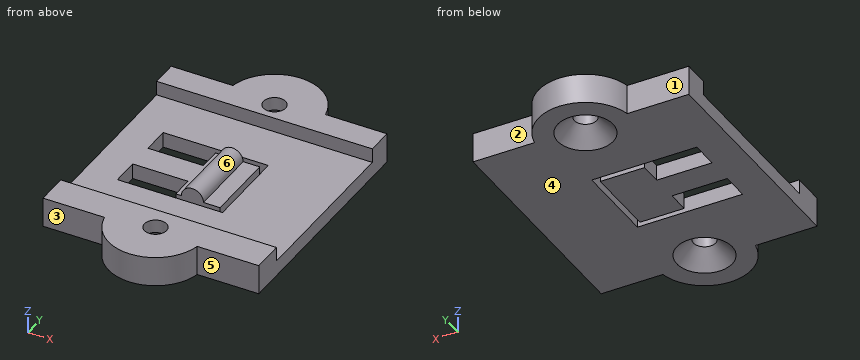
```python
from build123d import *

# Parameters (mm, degrees)
F1_DEPTH       = 5.4
F2_W           = 31.4
F2_H           = 2.6
F3_DEPTH       = 40
F4_W           = 2
F4_H           = 13
F6_D           = 4
F6_CSINK_D     = 10
F6_CSINK_ANGLE = 90


with BuildPart() as f1:
    # F0 (on Top) → F1 (new body)
    with BuildSketch(Plane.XY):
        with BuildLine():
            ThreePointArc((19.5610458605, 16.0277770907), (11.1944455951, 23.0277770907), (2.8278453298, 16.0277770907))
            Line((2.8278453298, 16.0277770907), (19.5610458605, 16.0277770907))
        make_face()
        with BuildLine():
            Line((19.5610458605, -25.9722229093), (2.8278453298, -25.9722229093))
            ThreePointArc((2.8278453298, -25.9722229093), (11.1944455951, -32.9722229093), (19.5610458605, -25.9722229093))
        make_face()
        with BuildLine():
            Line((2.8278453298, 16.0277770907), (-8.3055544049, 16.0277770907))
            Line((-8.3055544049, 16.0277770907), (-8.3055544049, -25.9722229093))
            Line((-8.3055544049, -25.9722229093), (2.8278453298, -25.9722229093))
            ThreePointArc((2.8278453298, -25.9722229093), (10.4414855216, -16.0056385255), (19.6944455951, -24.4722229093))
            ThreePointArc((19.6944455951, -24.4722229093), (19.6610299789, -25.2251829828), (19.5610458605, -25.9722229093))
            Line((19.5610458605, -25.9722229093), (30.6944455951, -25.9722229093))
            Line((30.6944455951, -25.9722229093), (30.6944455951, 16.0277770907))
            Line((30.6944455951, 16.0277770907), (19.5610458605, 16.0277770907))
            ThreePointArc((19.5610458605, 16.0277770907), (19.6610299789, 15.2807371642), (19.6944455951, 14.5277770907))
            ThreePointArc((19.6944455951, 14.5277770907), (10.4414855216, 6.0611927069), (2.8278453298, 16.0277770907))
        make_face()
        Polygon((7.6944455951, -7.4722229093), (7.6944455951, -2.4722229093), (-2.3055544049, -2.4722229093), (-2.3055544049, 2.5277770907), (7.6944455951, 2.5277770907), (16.6944455951, 2.5277770907), (16.6944455951, 1.5277770907), (16.6944455951, -11.4722229093), (16.6944455951, -12.4722229093), (7.6944455951, -12.4722229093), (-2.3055544049, -12.4722229093), (-2.3055544049, -7.4722229093), align=None, mode=Mode.SUBTRACT)
        with BuildLine():
            ThreePointArc((19.6944455951, -24.4722229093), (10.4414855216, -16.0056385255), (2.8278453298, -25.9722229093))
            Line((2.8278453298, -25.9722229093), (19.5610458605, -25.9722229093))
            ThreePointArc((19.5610458605, -25.9722229093), (19.6610299789, -25.2251829828), (19.6944455951, -24.4722229093))
        make_face()
        with BuildLine():
            Line((19.5610458605, 16.0277770907), (2.8278453298, 16.0277770907))
            ThreePointArc((2.8278453298, 16.0277770907), (10.4414855216, 6.0611927069), (19.6944455951, 14.5277770907))
            ThreePointArc((19.6944455951, 14.5277770907), (19.6610299789, 15.2807371642), (19.5610458605, 16.0277770907))
        make_face()
        Polygon((15.6944455951, 1.5277770907), (7.6944455951, 1.5277770907), (7.6944455951, -2.4722229093), (7.6944455951, -7.4722229093), (7.6944455951, -11.4722229093), (15.6944455951, -11.4722229093), align=None)
    extrude(amount=F1_DEPTH)

    # F2 (on face) → F3 (cut)
    with BuildSketch(Plane.YZ.offset(30.6944455951)):
        with Locations((-4.4722229093, 4.1)):
            Rectangle(F2_W, F2_H)
    extrude(amount=-F3_DEPTH, mode=Mode.SUBTRACT)

    # F4 (on face) → F5 (revolve)
    with BuildSketch(Plane.XY.offset(2.8)):
        with Locations((9.6944455951, -4.9722229093)):
            Rectangle(F4_W, F4_H)
    revolve(axis=Axis((10.6944455951, -4.9722229093, 2.8), (0, 1, 0)))

    # F6 (through all)
    with Locations(Plane(origin=(0, 0, 0), x_dir=(1, 0, 0), z_dir=(0, 0, -1))):
        with Locations((11.1944455951, 24.4722229093), (11.1944455951, -14.5277770907)):
            CounterSinkHole(F6_D / 2, F6_CSINK_D / 2, counter_sink_angle=F6_CSINK_ANGLE)


solid = f1.part
```
Read the model definition and answer for the solid it produces. Units are mm, in the model's axes. Face numbers are marked on the shaded views. A direction names the side the tool comes from. Round coordinates to 2 decimals unless told otherwise and drop trailing zeros. Write each loop counter-clockwise with the first axis right and the second up, starting at its lowest first coordinate (ties: lowest second). Pieces come first, ordered by that corner, then holes. Notation, with made-up numbers: (-3.5, 28.25) - (1.5, 28.25) arc R27 cw to (1.5, 64.25) - close; hole circle Ø4 at (-17, 85.5). An arc over 180 degrees is marked (long way). One line per item, written item: value.
Q1. Which of the six approach directions +Z, -Z, +X, -X, +Y, -Y give full straight-line access (tool end or side, diameter ignored) to the marked faces 1, 2 and 3?
The answers:
face 1: +Z, -Z, -X, +Y
face 2: +Z, -Z, +X, +Y
face 3: +Z, -Z, -X, -Y
Q2. For a pull along Y with two mould halves and no side action, classify the marked faces 4, 5 and 6 as pulls with the +Y half, pulls with the -Y half, needs draft (parallel to the pull), parting line crosses it, or undercut.
The answers:
face 4: needs draft
face 5: pulls with the -Y half
face 6: undercut
Q3. Straight lines are drawn through the part: line 1 (Y direction, x = 2.5, z = 0.4); line 2 (Y direction, x = -4, z = 4.1); line 3 (Y direction, x = 9, z = 0.65). For each, find the intervals that lie inside material, in ascending order. Write a range as from..to.
The answers:
line 1: y = -25.97..-12.47, -7.47..-2.47, 2.53..16.03
line 2: y = -25.97..-20.17, 11.23..16.03
line 3: y = -32.68..-28.23, -20.72..-12.47, -11.47..1.53, 2.53..10.77, 18.28..22.74
Q4. Each of these flat-tipped pins is pushed along its axis until it touches: P1, Ø1, axis at x = 7, y = -13.5, coming from the +Z side; P2, Ø1.6, axis at x = 26, z = 3.5, coming from the +Y side; P3, Ø3, axis at x = 3.5, z = 1, coming from the -Y side. Where does it stop, or does it pass through?
The answers:
P1: stops at z = 2.8
P2: stops at y = 16.03
P3: stops at y = -30.29
Q5. Find section D-D (y = 6). Determine the outline of the cut face in (x, z).
The answers:
outline: (-8.31, 0) - (30.69, 0) - (30.69, 2.8) - (-8.31, 2.8) - close
Q6. Find section B-B (x = 1). Determine the outline of the cut face in (y, z), and give its area (3 significant figures).
The answers:
outline: (-25.97, 0) - (-12.47, 0) - (-12.47, 2.8) - (-20.17, 2.8) - (-20.17, 5.4) - (-25.97, 5.4) - close; (-7.47, 0) - (-2.47, 0) - (-2.47, 2.8) - (-7.47, 2.8) - close; (2.53, 0) - (16.03, 0) - (16.03, 5.4) - (11.23, 5.4) - (11.23, 2.8) - (2.53, 2.8) - close
area: 117 mm2
Q7. Find section A-A (y = -8.5). Determine the outline of the cut face in (x, z).
The answers:
outline: (-8.31, 0) - (-2.31, 0) - (-2.31, 2.8) - (-8.31, 2.8) - close; (7.69, 0) - (15.69, 0) - (15.69, 2.8) - (12.69, 2.8) arc R2 ccw to (8.69, 2.8) - (7.69, 2.8) - close; (16.69, 0) - (30.69, 0) - (30.69, 2.8) - (16.69, 2.8) - close
Q8. Find section C-C (x = 28.5). Determine the outline of the cut face in (y, z), and give its area (3 significant figures).
The answers:
outline: (-25.97, 0) - (16.03, 0) - (16.03, 5.4) - (11.23, 5.4) - (11.23, 2.8) - (-20.17, 2.8) - (-20.17, 5.4) - (-25.97, 5.4) - close
area: 145 mm2
